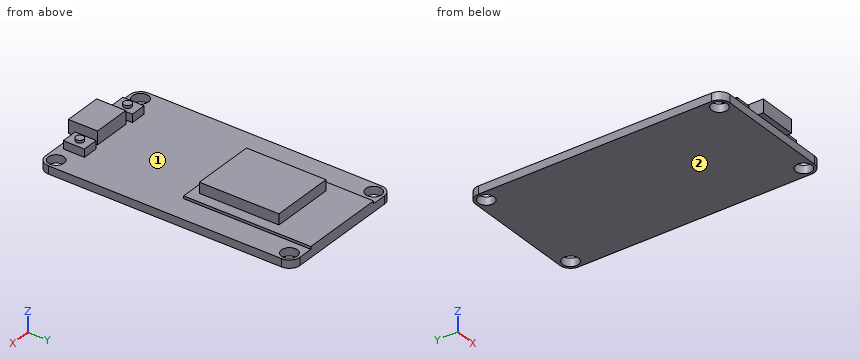
from build123d import *

# Parameters (mm, degrees)
SKETCH1_W              = 25.5
SKETCH1_H              = 48
PCB_DEPTH              = 1.5
FILLET1_R              = 2
SCREW_HOLES_DEPTH      = 28.217870967
SCREW_HOLES_DEPTH_BACK = 28.217870967
SKETCH2_R              = 1.5
SKETCH3_W              = 16
SKETCH3_H              = 24
ESP_PCB_DEPTH          = 0.5
SKETCH4_W              = 12
SKETCH4_H              = 15
RF_CASING_DEPTH        = 2
SKETCH5_W              = 7.2
SKETCH5_H              = 5.5
USB_PORT_DEPTH         = 2.5
SKETCH6_W              = 3
SKETCH6_H              = 4
BUTTON_BOTTOM_DEPTH    = 1.5
SKETCH7_R              = 0.75
BUTTON_TOP_DEPTH       = 0.5


with BuildPart() as part:
    # Sketch1 → PCB (new body)
    with BuildSketch(Plane.XY):
        Rectangle(SKETCH1_W, SKETCH1_H)
    extrude(amount=PCB_DEPTH)

    # Fillet1
    fillet1_edges = [part.edges().sort_by_distance(p)[0] for p in [
        (12.75, -24, 0.75),
        (-12.75, -24, 0.75),
        (-12.75, 24, 0.75),
        (12.75, 24, 0.75),
    ]]
    fillet(fillet1_edges, radius=FILLET1_R)

    # Sketch2 → Screw holes (cut, two sides: drawn at the far end of the back side and taken through both)
    with BuildSketch(Plane.XY.offset(1.5).offset(-SCREW_HOLES_DEPTH_BACK)):
        with Locations((-10.75, 22)):
            Circle(SKETCH2_R)
        with Locations((10.75, 22)):
            Circle(SKETCH2_R)
        with Locations((10.75, -22)):
            Circle(SKETCH2_R)
        with Locations((-10.75, -22)):
            Circle(SKETCH2_R)
    extrude(amount=SCREW_HOLES_DEPTH + SCREW_HOLES_DEPTH_BACK, mode=Mode.SUBTRACT)

    # Sketch3 → ESP PCB (add)
    with BuildSketch(Plane.XY.offset(1.5)):
        with Locations((0, 12)):
            Rectangle(SKETCH3_W, SKETCH3_H)
    extrude(amount=ESP_PCB_DEPTH)

    # Sketch4 → RF Casing (add)
    with BuildSketch(Plane.XY.offset(2)):
        with Locations((0, 9)):
            Rectangle(SKETCH4_W, SKETCH4_H)
    extrude(amount=RF_CASING_DEPTH)

    # Sketch5 → USB Port (add)
    with BuildSketch(Plane.XY.offset(1.5)):
        with Locations((0, -22.25)):
            Rectangle(SKETCH5_W, SKETCH5_H)
    extrude(amount=USB_PORT_DEPTH)

    # Sketch6 → Button Bottom (add)
    with BuildSketch(Plane.XY.offset(1.5)):
        with Locations((-6.1, -21)):
            Rectangle(SKETCH6_W, SKETCH6_H)
        with Locations((6.1, -21)):
            Rectangle(SKETCH6_W, SKETCH6_H)
    extrude(amount=BUTTON_BOTTOM_DEPTH)

    # Sketch7 → Button Top (add)
    with BuildSketch(Plane.XY.offset(3)):
        with Locations((-6.1, -21)):
            Circle(SKETCH7_R)
        with Locations((6.1, -21)):
            Circle(SKETCH7_R)
    extrude(amount=BUTTON_TOP_DEPTH)


solid = part.part
Part model, mm, in its own coordinate system. Face numbers are marked on the shaded views. Coordinates: 2 decimals unless noted, no trailing zeros. Loops run counter-clockwise (first coordinate to the right, second up) from the corner with the lowest first, then second, coordinate; pieces in that order, holes last. Notation, with made-up numbers: M 46,4 L 74,4 A18 ccw 74,36 Z; hole C -20,31.25 d5. An arc over 180 degrees is marked long. Use a Markdown table: item, result. Add a question column.
Q1. Cut at D-D (x = 10.25). Write the cut outline in (y, z).
Q2. Pin check, flat tips, straight feed: P1, Ø1.5, axis at x = -6.5, y = -20.5, coming from the +Z side; P2, Ø0.6, axis at y = 8.5, z = 3, coming from the +X side; P3, Ø0.8, axis at x = -6, z = 2, coming from the -Y side. Stop position of each tip, or through.
Q3. Cut at B-B (y = -21). Give the number of separate pieces and of enclosed holes in the cut face, and give its area (3 significant figures).
Q4. Mould opens along Y. For the marked faces 1 and 2 say: +Y half, -Y half, draft (parallel to the pull), parting line (faces both ways), or undercut.
Q5. Cut at A-A (z = 0.9). Write the cut outline in (x, y).
Q6. Probe L1, parallel to X at y = -22, z = 0.85; L2, parallel to Y at x = -10.75, z = 0.5; L3, parallel to X at y = -20.5, z = 2.65. List the from-to ranges inside material, lowest first.
Q7. Cut at C-C (x = -2.25). Write the cut outline in (y, z).
Worked out:
| question | item | result |
|---|---|---|
| 1 | outline | M -24,0 L -23.41,0 L -23.41,1.5 L -24,1.5 Z; M -20.59,0 L 20.59,0 L 20.59,1.5 L -20.59,1.5 Z; M 23.41,0 L 24,0 L 24,1.5 L 23.41,1.5 Z |
| 2 | P1 | stops at z = 3.5 |
| 2 | P2 | stops at x = 6 |
| 2 | P3 | stops at y = -23 |
| 3 | separate pieces | 3 |
| 3 | enclosed holes | 0 |
| 3 | area | 60.0 mm2 |
| 4 | face 1 | undercut |
| 4 | face 2 | draft |
| 5 | outline | M -12.75,-22 A2 ccw -10.75,-24 L 10.75,-24 A2 ccw 12.75,-22 L 12.75,22 A2 ccw 10.75,24 L -10.75,24 A2 ccw -12.75,22 Z; hole C -10.75,-22 d3; hole C -10.75,22 d3; hole C 10.75,-22 d3; hole C 10.75,22 d3 |
| 6 | L1 | x = -12.75 to -12.25, -9.25 to 9.25, 12.25 to 12.75 |
| 6 | L2 | y = -24 to -23.5, -20.5 to 20.5, 23.5 to 24 |
| 6 | L3 | x = -7.6 to -4.6, -3.6 to 3.6, 4.6 to 7.6 |
| 7 | outline | M -25,1.5 L -24,1.5 L -24,0 L 24,0 L 24,2 L 16.5,2 L 16.5,4 L 1.5,4 L 1.5,2 L 0,2 L 0,1.5 L -19.5,1.5 L -19.5,4 L -25,4 Z |
